Model file for the job. Use its own axes, mm. Give positions to 0.01 mm unless a question says otherwise; leave off trailing zeros. Order: outer loops, then holes, each group sorted by start corner. A loop starts at its lowest first (then second) coordinate and runs counter-clockwise, first axis right, second up. Notation, with made-up numbers: M -20,29 L 35,29 A22 cw 35,50 Z; hole C 86.25,-2.75 d1. An arc over 180 degrees is marked long. Return JSON: item names as keys, results as strings. Group by question number.
1. Wall check: probe 1 along Z at (x, y) = (0, -5.5); probe 2 along Z at (x, y) = (1.75, -1.5); probe 3 along X at (y, z) = (-3.75, -3.75). Give the ranges that are in metal, low to high. Write a range as [from, to].
2. Slice it at A-A on z = -2. List the corners of the cut face in (x, y), then the cut area to 3 significant figures.
3. Slice it at D-D on y = -0.5. List the corners of the cut face in (x, z).
4. Slice it at B-B on y = -4.25. List the corners of the cut face in (x, z).
5. Slice it at C-C on x = 0.25. List the corners of the cut face in (y, z), then the cut area to 3 significant figures.
6. Pin check, flat tips, straight feed: pin 1 (3 mm diameter, centred on y = -2.5, z = 0, fed in from +X); pin 2 (1.5 mm diameter, centred on y = -3, z = -3, fed in from -X); pin 3 (4 mm diameter, centred on y = -6, z = 4, fed in from +X); pin 4 (2 mm diameter, centred on x = -2.5, y = -4, fed in from -Z). Stop position of each tip, or through.
7. Two-plate mould, pull along X, no slides. Class faces 1 (the face through (5.34, -3.46, -3.11)), 2 (the face through (4, 0, 2)), 3 (the face through (-2.285, -3.549, -3.584)): released by +X, released by -X, zero draft, split by the parting line, or undercut.
from build123d import *

# Parameters (mm, degrees)
F1_DEPTH = 7
F2_SIZE  = 1
F3_SIZE  = 1
F4_D     = 8.5


with BuildPart() as f1:
    # F0 (on Front) → F1 (new body)
    with BuildSketch(Plane.XZ):
        with BuildLine():
            ThreePointArc((5.3637862302, -3.0659549776), (5.9711339811, -1.5861404815), (6.178210311, 0))
            ThreePointArc((6.178210311, 0), (5.9642239682, 1.6119290011), (5.3370880527, 3.1121975781))
            ThreePointArc((5.3370880527, 3.1121975781), (3.0659549821, 5.3637862276), (-0.0266982871, 6.1781526243))
            ThreePointArc((-0.0266982871, 6.1781526243), (-3.1121976822, 5.337087992), (-5.3637862362, 3.065954967))
            ThreePointArc((-5.3637862362, 3.065954967), (-6.1781526243, -0.0266982826), (-5.3370879532, -3.1121977488))
            ThreePointArc((-5.3370879532, -3.1121977488), (-3.0659548546, -5.3637863004), (0.026698383, -6.1781526239))
            ThreePointArc((0.026698383, -6.1781526239), (3.1121977184, -5.3370879709), (5.3637862302, -3.0659549776))
        make_face()
        with BuildLine():
            ThreePointArc((5.3370880527, 3.1121975781), (5.9642239682, 1.6119290011), (6.178210311, 0))
            ThreePointArc((6.178210311, 0), (5.9711339811, -1.5861404815), (5.3637862302, -3.0659549776))
            Line((5.3637862302, -3.0659549776), (7.1339161613, 0.0308285647))
            Line((7.1339161613, 0.0308285647), (5.3370880527, 3.1121975781))
        make_face()
        with BuildLine():
            ThreePointArc((-0.0266982871, 6.1781526243), (3.0659549821, 5.3637862276), (5.3370880527, 3.1121975781))
            Line((5.3370880527, 3.1121975781), (3.5402597604, 6.1935669065))
            Line((3.5402597604, 6.1935669065), (-0.0266982871, 6.1781526243))
        make_face()
        with BuildLine():
            Line((3.5936564009, -6.1627383418), (5.3637862302, -3.0659549776))
            ThreePointArc((5.3637862302, -3.0659549776), (3.1121977184, -5.3370879709), (0.026698383, -6.1781526239))
            Line((0.026698383, -6.1781526239), (3.5936564009, -6.1627383418))
        make_face()
        with BuildLine():
            ThreePointArc((-5.3637862362, 3.065954967), (-3.1121976822, 5.337087992), (-0.0266982871, 6.1781526243))
            Line((-0.0266982871, 6.1781526243), (-3.5936564009, 6.1627383418))
            Line((-3.5936564009, 6.1627383418), (-5.3637862362, 3.065954967))
        make_face()
        with BuildLine():
            Line((-3.5402597604, -6.1935669065), (0.026698383, -6.1781526239))
            ThreePointArc((0.026698383, -6.1781526239), (-3.0659548546, -5.3637863004), (-5.3370879532, -3.1121977488))
            Line((-5.3370879532, -3.1121977488), (-3.5402597604, -6.1935669065))
        make_face()
        with BuildLine():
            ThreePointArc((-5.3370879532, -3.1121977488), (-6.1781526243, -0.0266982826), (-5.3637862362, 3.065954967))
            Line((-5.3637862362, 3.065954967), (-7.1339161613, -0.0308285647))
            Line((-7.1339161613, -0.0308285647), (-5.3370879532, -3.1121977488))
        make_face()
    extrude(amount=F1_DEPTH)

    # F2
    f2_edges = [f1.edges().sort_by_distance(p)[0] for p in [
        (-5.363786, -7, 3.065955),
        (-0.026698, -7, 6.178153),
        (5.337088, -7, 3.112198),
        (5.363786, -7, -3.065955),
        (0.026698, -7, -6.178153),
        (-5.337088, -7, -3.112198),
    ]]
    chamfer(f2_edges, length=F2_SIZE)

    # F3
    f3_edges = [f1.edges().sort_by_distance(p)[0] for p in [
        (5.337088, 0, 3.112198),
        (-0.026698, 0, 6.178153),
        (-5.363786, 0, 3.065955),
        (-5.337088, 0, -3.112198),
        (0.026698, 0, -6.178153),
        (5.363786, 0, -3.065955),
    ]]
    chamfer(f3_edges, length=F3_SIZE)

    # F4 (through all)
    with Locations(Plane(origin=(0, 0, 0), x_dir=(1, 0, 0), z_dir=(0, 1, 0))):
        with Locations((0, 0)):
            Hole(F4_D / 2)


solid = f1.part
Result:
{
 "1": {"probe 1": "z = [-6.18, -4.25], [4.25, 6.18]", "probe 2": "z = [-6.17, -3.87], [3.87, 6.19]", "probe 3": "x = [-4.97, -2], [2, 4.97]"},
 "2": {"outline": "M -5.99,-6 L -4.83,-7 L -3.75,-7 L -3.75,0 L -4.83,0 L -5.99,-1 Z; M 3.75,-7 L 4.82,-7 L 5.97,-6 L 5.97,-1 L 4.82,0 L 3.75,0 Z", "area": "28.9 mm2"},
 "3": {"outline": "M -6.56,-0.03 L -3.25,-5.69 L 3.3,-5.66 L 6.56,0.03 L 3.25,5.69 L -3.3,5.66 Z; hole C 0,0 d8.5"},
 "4": {"outline": "M -7.13,-0.03 L -3.54,-6.19 L 3.59,-6.16 L 7.13,0.03 L 3.54,6.19 L -3.59,6.16 Z; hole C 0,0 d8.5"},
 "5": {"outline": "M -7,-5.18 L -6,-6.18 L -1,-6.18 L 0,-5.18 L 0,-4.24 L -7,-4.24 Z; M -7,4.24 L 0,4.24 L 0,5.18 L -1,6.18 L -6,6.18 L -7,5.18 Z", "area": "25.1 mm2"},
 "6": {"pin 1": "stops at x = 7.13", "pin 2": "stops at x = -5.84", "pin 3": "stops at x = 5.99", "pin 4": "stops at z = -6.19"},
 "7": {"face 1": "released by +X", "face 2": "zero draft", "face 3": "undercut"}
}
